Geometry: final body of the model. Coordinates: model frame, mm. Face numbers are marked on the shaded views. A direction names the side the tool comes from. Round coordinates to 2 decimals unless told otherwise and drop trailing zeros. Order: outer loops, then holes, each group sorted by start corner. A loop starts at its lowest first (then second) coordinate and runs counter-clockwise, first axis right, second up. Notation, with made-up numbers: M 38.25,56 L 54.25,56 A30 ccw 54.25,80 Z; hole C -11.75,58 d9. An arc over 180 degrees is marked long. Put each result on its own line as item: value. Start each with the question number.
1) First-contact query: P1, Ø2, axis at x = 46.5, z = 59.5, coming from the +Y side (3 decimals); P2, Ø3.5, axis at x = 27.47, z = 66.46, coming from the -Y side; P3, Ø12, axis at x = -70.5, y = 48.5, coming from the +Z side (3 decimals); P4, Ø2.5, axis at x = 36, y = 81, coming from the +Z side. Flat tips, straight axial feed; report the tip coordinate or a pass-through.
2) Section A-A, the plane z = 42.5. Return loops of the section in (x, y) (3 decimals).
3) Draft query along Y for the marked faces 3, 4 and 5. Return one class per face: pulls with the +Y half, pulls with the -Y half, needs draft (parallel to the pull), parting line crosses it, or undercut.
4) Section C-C, the plane y = -31. Return loops of the section in (x, z) (3 decimals), then the cut area to 3 significant figures.
5) Access query for the marked faces 1 and 2. Directions: +Z, -Z, +X, -X, +Y, -Y. A direction counts if a zero-diameter tool reaches every point of the face in a straight line with its end or side. Return the directions, or none.
6) Section B-B, the plane x = -54.5. Return loops of the section in (y, z) (3 decimals), then the cut area to 3 significant figures.
7) Material intervals for probe 1 along X at (y, z) = (62.5, 67); probe 2 along Z at (x, y) = (-103, -12); probe 3 along Y at (x, z) = (62, 43.5) (3 decimals), sorted ascending. Write a range as [from, to].
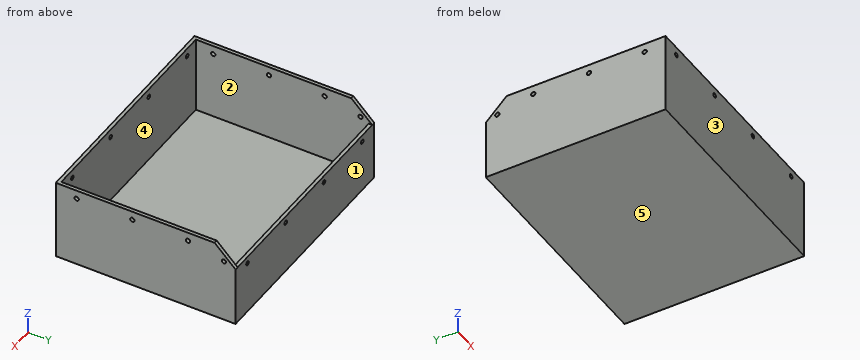
from build123d import *

# Parameters (mm, degrees)
SKETCH2_W                = 211.751333334
SKETCH2_H                = 164
BOSS_EXTRUDE1_DEPTH      = 74.083333333
CUT_EXTRUDE7_DEPTH       = 70.90833333
CUT_EXTRUDE9_REACH       = 240.853
CUT_EXTRUDE10_DEPTH      = 3.175
SKETCH14_W               = 205.401333334
SKETCH14_H               = 3.175
CUT_EXTRUDE11_DEPTH      = 3.175
CUT_EXTRUDE12_DEPTH      = 239.853443446
CUT_EXTRUDE12_DEPTH_BACK = 3.175
SKETCH16_R               = 2
CUT_EXTRUDE13_DEPTH      = 239.853443446
LPATTERN1_COUNT          = 3
LPATTERN1_PITCH          = 50.8
CUT_EXTRUDE14_REACH      = 210.792
SKETCH18_R               = 2
LPATTERN2_COUNT          = 4
LPATTERN2_PITCH          = 58.42
CUT_EXTRUDE15_REACH      = 210.792
SKETCH19_R               = 2
LPATTERN3_COUNT          = 4
LPATTERN3_PITCH          = 58.42
SKETCH20_R               = 2
CUT_EXTRUDE16_DEPTH      = 239.853443446


with BuildPart() as part:
    # Sketch2 → Boss-Extrude1 (new body)
    with BuildSketch(Plane.XY):
        Rectangle(SKETCH2_W, SKETCH2_H)
    extrude(amount=BOSS_EXTRUDE1_DEPTH)

    # Sketch9 → Cut-Extrude7 (cut)
    with BuildSketch(Plane.XY.offset(74.083333333)):
        Polygon((-102.700666667, 62.95), (-102.700666667, -47.748173381), (-102.700666667, -78.825), (-61.266487403, -78.825), (102.700666667, -78.825), (102.700666667, -21.962957065), (102.700666667, 78.825), (-87.76182231, 78.825), (-102.700666667, 78.825), align=None)
    extrude(amount=-CUT_EXTRUDE7_DEPTH, mode=Mode.SUBTRACT)

    # Sketch11 → Cut-Extrude9 (cut, up to next)
    with BuildSketch(Plane.ZY.offset(105.875666667), mode=Mode.PRIVATE) as cut_extrude9_sk1:
        Polygon((58.208333333, 78.825), (74.083333333, 62.95), (74.083333333, 82), (58.208333333, 82), (58.208333333, 79.62382388), align=None)
    cut_extrude9_tool1 = extrude(cut_extrude9_sk1.sketch, amount=-CUT_EXTRUDE9_REACH, mode=Mode.PRIVATE) & part.part
    add(cut_extrude9_tool1.solids().sort_by_distance((-105.875667, 75.49881, 68.035714))[0], mode=Mode.SUBTRACT)

    # Sketch13 → Cut-Extrude10 (cut)
    with BuildSketch(Plane.ZY.offset(105.875666667)):
        Polygon((58.208333333, 78.825), (55.033333333, 82), (58.208333333, 82), align=None)
    extrude(amount=-CUT_EXTRUDE10_DEPTH, mode=Mode.SUBTRACT)

    # Sketch14 → Cut-Extrude11 (cut)
    with BuildSketch(Plane.XY.offset(58.208333333)):
        with Locations((0, 80.4125)):
            Rectangle(SKETCH14_W, SKETCH14_H)
    extrude(amount=-CUT_EXTRUDE11_DEPTH, mode=Mode.SUBTRACT)

    # Sketch15 → Cut-Extrude12 (cut, two sides: drawn at the far end of the back side and taken through both)
    with BuildSketch(Plane(origin=(105.875666667, 0, 0), x_dir=(0, 0, -1), z_dir=(1, 0, 0)).offset(-CUT_EXTRUDE12_DEPTH_BACK)):
        Polygon((-58.208333333, 79.215720039), (-58.208333333, 78.825), (-55.033333333, 82), (-58.208333333, 82), align=None)
    extrude(amount=CUT_EXTRUDE12_DEPTH + CUT_EXTRUDE12_DEPTH_BACK, mode=Mode.SUBTRACT)

    # Sketch16 → Cut-Extrude13 (cut, through all)
    with BuildSketch(Plane.ZY.offset(105.875666667)):
        with Locations((65.955333333, -62.95)):
            Circle(SKETCH16_R)
    cut_extrude13 = extrude(amount=-CUT_EXTRUDE13_DEPTH, mode=Mode.SUBTRACT)

    # LPattern1: Cut-Extrude13 ×3
    with Locations(*[(0, i * LPATTERN1_PITCH, 0) for i in range(1, LPATTERN1_COUNT)]):
        add(cut_extrude13, mode=Mode.SUBTRACT)

    # Sketch18 → Cut-Extrude14 (cut, up to next)
    with BuildSketch(Plane.XZ.offset(82), mode=Mode.PRIVATE) as cut_extrude14_sk1:
        with Locations(Location((-89.365666667, 66.463333333, 0), (0, 0, 270))):
            Circle(SKETCH18_R)
    cut_extrude14_tool1 = extrude(cut_extrude14_sk1.sketch, amount=-CUT_EXTRUDE14_REACH, mode=Mode.PRIVATE) & part.part
    cut_extrude14 = cut_extrude14_tool1.solids().sort_by_distance((-89.365667, -82, 66.463333))[0]
    add(cut_extrude14, mode=Mode.SUBTRACT)

    # LPattern2: Cut-Extrude14 ×4
    with Locations(*[(i * LPATTERN2_PITCH, 0, 0) for i in range(1, LPATTERN2_COUNT)]):
        add(cut_extrude14, mode=Mode.SUBTRACT)

    # Sketch19 → Cut-Extrude15 (cut, up to next)
    with BuildSketch(Plane(origin=(0, 82, 0), x_dir=(1, 0, 0), z_dir=(0, 1, 0)), mode=Mode.PRIVATE) as cut_extrude15_sk1:
        with Locations(Location((-87.587666667, -48.683333333, 0), (0, 0, 270))):
            Circle(SKETCH19_R)
    cut_extrude15_tool1 = extrude(cut_extrude15_sk1.sketch, amount=-CUT_EXTRUDE15_REACH, mode=Mode.PRIVATE) & part.part
    cut_extrude15 = cut_extrude15_tool1.solids().sort_by_distance((-87.587667, 82, 48.683333))[0]
    add(cut_extrude15, mode=Mode.SUBTRACT)

    # LPattern3: Cut-Extrude15 ×4
    with Locations(*[(i * LPATTERN3_PITCH, 0, 0) for i in range(1, LPATTERN3_COUNT)]):
        add(cut_extrude15, mode=Mode.SUBTRACT)

    # Sketch20 → Cut-Extrude16 (cut, through all)
    with BuildSketch(Plane.ZY.offset(105.875666667)):
        with Locations((58.805040904, 71.403297777)):
            Circle(SKETCH20_R)
    extrude(amount=-CUT_EXTRUDE16_DEPTH, mode=Mode.SUBTRACT)


solid = part.part
Result sheet:
1. P1: stops at y = -78.825
1. P2: passes through
1. P3: stops at z = 3.175
1. P4: stops at z = 55.03
2. outline: M -105.876,-82 L 105.876,-82 L 105.876,82 L -105.876,82 Z; hole M -102.701,-78.825 L 102.701,-78.825 L 102.701,78.825 L -102.701,78.825 Z
3. face 3: pulls with the -Y half
3. face 4: undercut
3. face 5: needs draft
4. outline: M -105.876,0 L 105.876,0 L 105.876,74.083 L 102.701,74.083 L 102.701,3.175 L -102.701,3.175 L -102.701,74.083 L -105.876,74.083 Z
4. area: 1,120 mm2
5. face 1: +Z, -Z, +X, -X, +Y
5. face 2: +Z
6. outline: M -82,0 L 82,0 L 82,55.033 L 78.825,55.033 L 78.825,3.175 L -78.825,3.175 L -78.825,74.083 L -82,74.083 Z
6. area: 910 mm2
7. probe 1: x = [-105.88, -102.7], [102.7, 105.88]
7. probe 2: z = [0, 63.96], [67.95, 74.08]
7. probe 3: y = [-82, -78.825], [78.825, 82]
